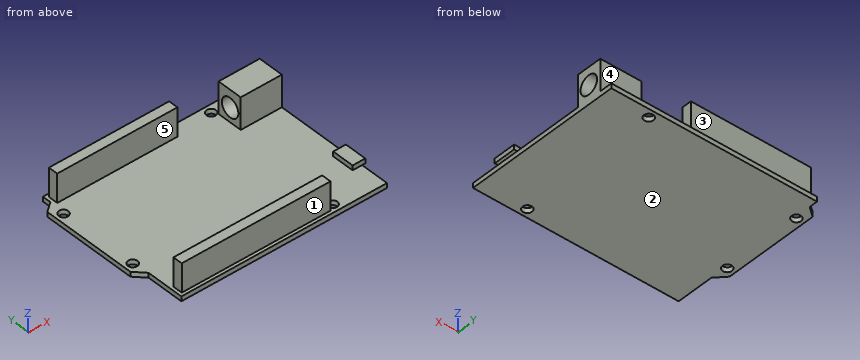
from build123d import *

# Parameters (mm, degrees)
F0_R     = 1.5
F1_DEPTH = 1.5
F2_W     = 38
F2_H     = 3
F2_W_2   = 47
F3_DEPTH = 9
F4_W     = 4
F4_H     = 7
F5_DEPTH = 1.5
F6_W     = 8
F6_H     = 1.5
F6_H_2   = 10
F6_R     = 3
F7_DEPTH = 13


with BuildPart() as f1:
    # F0 (on Top) → F1 (new body)
    with BuildSketch(Plane.XY):
        Polygon((15.091755, -23.95556), (15.091755, 26.04444), (-49.908245, 26.04444), (-49.908245, 23.392303), (-52.908245, 21.04444), (-52.908245, -8.95556), (-49.908245, -12.139853), (-49.908245, -23.95556), align=None)
        with Locations((-50.408245, -6.95556)):
            Circle(F0_R, mode=Mode.SUBTRACT)
        with Locations((0.091755, -21.45556)):
            Circle(F0_R, mode=Mode.SUBTRACT)
        with Locations((-50.408245, 18.04444)):
            Circle(F0_R, mode=Mode.SUBTRACT)
        with Locations((1.091755, 23.54444)):
            Circle(F0_R, mode=Mode.SUBTRACT)
    extrude(amount=F1_DEPTH)

    # F2 (on face) → F3 (join)
    with BuildSketch(Plane.XY.offset(1.5)):
        with Locations((-29.908245, 23.54444)):
            Rectangle(F2_W, F2_H)
        with Locations((-25.408245, -21.45556)):
            Rectangle(F2_W_2, F2_H)
    extrude(amount=F3_DEPTH)

    # F4 (on face) → F5 (join)
    with BuildSketch(Plane.XY.offset(1.5)):
        with Locations((14.091755, -11.45556)):
            Rectangle(F4_W, F4_H)
    extrude(amount=F5_DEPTH)

    # F6 (on face) → F7 (join)
    with BuildSketch(Plane.YZ.offset(15.091755)):
        with Locations((18.04444, 0.75)):
            Rectangle(F6_W, F6_H)
        with Locations((18.04444, 6.5)):
            Rectangle(F6_W, F6_H_2)
        with Locations((17.887879, 6)):
            Circle(F6_R, mode=Mode.SUBTRACT)
    extrude(amount=-F7_DEPTH)


solid = f1.part
Source: CAD feature listing. Evaluate the final solid. Frame: model axes, mm. Face numbers are marked on the shaded views. A direction names the side the tool comes from. Give positions to 0.01 mm unless a question says otherwise; leave off trailing zeros. Write each loop counter-clockwise with the first axis right and the second up, starting at its lowest first coordinate (ties: lowest second). Pieces come first, ordered by that corner, then holes. Notation, with made-up numbers: (-27.75, 15) -> (-21.75, 15) arc R27 cw to (-21.75, 32) -> close; hole circle Ø8 at (36.25, 55.25). An arc over 180 degrees is marked (long way). Return JSON: item names as keys, results as strings. Group by question number.
1. Section D-D, the plane y = -10.5. Output: boundary loops of the cut face in (x, z), then the cut area to 3 significant figures.
2. Section A-A, the plane x = 9. Output: boundary loops of the cut face in (y, z).
3. Section B-B, the plane z = 6. Output: boundary loops of the cut face in (x, y).
4. Access query for the marked faces 1, 2, 3, 4 and 5. Directions: +Z, -Z, +X, -X, +Y, -Y. A direction counts if a zero-diameter tool reaches every point of the face in a straight line with its end or side. Return the directions, or none.
5. Pin query (flat end, axial travel): pin 1 Ø6.5 at (y, z) = (18, 7.5) entering from -X; pin 2 Ø2.5 at (x, z) = (-31, 5) entering from +Y; pin 3 Ø0.9 at (y, z) = (-21, 4) entering from +X; pin 4 Ø1.8 at (x, y) = (-50.41, -6.96) entering from +Z. Return the tip coordinate at first contact, or that it passes through.
6. Material intervals for line 1 (Y direction, x = -32, z = 6.25); line 2 (Z direction, x = -3.5, y = 11.5); line 3 (Y direction, x = 4.5, z = 7.5), sorted ascending. Write a range as from..to.
7. Section C-C, the plane x = -24. Output: boundary loops of the cut face in (y, z).
Determined:
{
 "1": {"outline": "(-51.45, 0) -> (15.09, 0) -> (15.09, 1.5) -> (16.09, 1.5) -> (16.09, 3) -> (12.09, 3) -> (12.09, 1.5) -> (-51.45, 1.5) -> close", "area": "106 mm2"},
 "2": {"outline": "(-23.96, 0) -> (26.04, 0) -> (26.04, 1.5) -> (22.04, 1.5) -> (22.04, 11.5) -> (14.04, 11.5) -> (14.04, 1.5) -> (-23.96, 1.5) -> close; hole circle Ø6 at (17.89, 6)"},
 "3": {"outline": "(-48.91, -22.96) -> (-1.91, -22.96) -> (-1.91, -19.96) -> (-48.91, -19.96) -> close; (-48.91, 22.04) -> (-10.91, 22.04) -> (-10.91, 25.04) -> (-48.91, 25.04) -> close; (2.09, 14.04) -> (15.09, 14.04) -> (15.09, 14.89) -> (2.09, 14.89) -> close; (2.09, 20.89) -> (15.09, 20.89) -> (15.09, 22.04) -> (2.09, 22.04) -> close"},
 "4": {"face 1": "+Z, +X, -X, -Y", "face 2": "-Z, +X, -X, +Y, -Y", "face 3": "+Z, +X, -X, +Y", "face 4": "+Z, +X, +Y", "face 5": "+Z, -X"},
 "5": {"pin 1": "stops at x = 2.09", "pin 2": "stops at y = 25.04", "pin 3": "stops at x = -1.91", "pin 4": "passes through"},
 "6": {"line 1": "y = -22.96..-19.96, 22.04..25.04", "line 2": "z = 0..1.5", "line 3": "y = 14.04..15.29, 20.49..22.04"},
 "7": {"outline": "(-23.96, 0) -> (26.04, 0) -> (26.04, 1.5) -> (25.04, 1.5) -> (25.04, 10.5) -> (22.04, 10.5) -> (22.04, 1.5) -> (-19.96, 1.5) -> (-19.96, 10.5) -> (-22.96, 10.5) -> (-22.96, 1.5) -> (-23.96, 1.5) -> close"}
}
